Source: CAD feature listing. Evaluate the final solid. Frame: model axes, mm. Face numbers are marked on the shaded views. A direction names the side the tool comes from. Give positions to 0.01 mm unless a question says otherwise; leave off trailing zeros. Loops run counter-clockwise (first coordinate to the right, second up) from the corner with the lowest first, then second, coordinate; pieces in that order, holes last. Notation, with made-up numbers: M -25.75,-32 L 17.25,-32 A14 ccw 17.25,-5 Z; hole C -3.5,13.25 d5. An arc over 180 degrees is marked long. Answer in a Markdown table with one row per item.
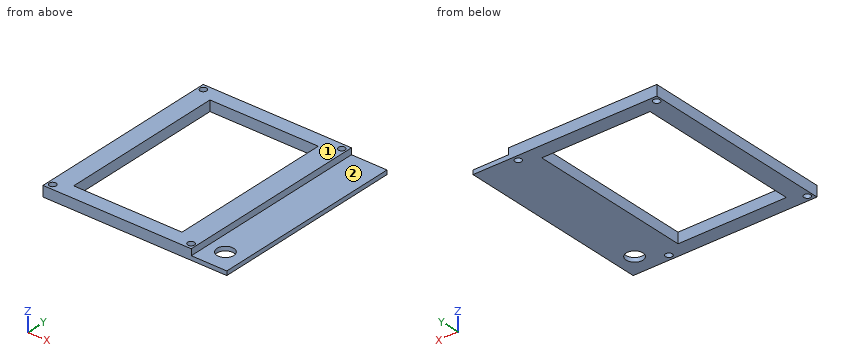
```python
from build123d import *

# Parameters (mm, degrees)
SKETCH_1_W          = 71
SKETCH_1_H          = 93
SKETCH_1_R          = 1.6
SKETCH_1_W_2        = 51
SKETCH_1_H_2        = 78.2
EXTRUDE_1_DEPTH     = 5
SKETCH_2_W          = 71
SKETCH_2_H          = 93
SKETCH_2_W_2        = 70.5
SKETCH_2_H_2        = 92.5
CUT_EXTRUDE_1_DEPTH = 6
SKETCH_3_W          = 51.5
SKETCH_3_H          = 78.7
SKETCH_3_W_2        = 51
SKETCH_3_H_2        = 78.2
CUT_EXTRUDE_2_DEPTH = 6
SKETCH_5_W          = 27
SKETCH_5_H          = 92.5
SKETCH_5_R          = 1.6
EXTRUDE_3_DEPTH     = 2
SKETCH_7_R          = 4
CUT_EXTRUDE_3_DEPTH = 6


with BuildPart() as part:
    # Эскиз1 → Бобышка-Вытянуть1 (new body)
    with BuildSketch(Plane(origin=(0, 0, 92.662297423), x_dir=(-1, 0, 0), z_dir=(0, 0, -1))):
        with Locations((-39.5, 51)):
            Rectangle(SKETCH_1_W, SKETCH_1_H)
        with Locations((-6.6, 7.5)):
            Circle(SKETCH_1_R, mode=Mode.SUBTRACT)
        with Locations((-72.4, 7.5)):
            Circle(SKETCH_1_R, mode=Mode.SUBTRACT)
        with Locations((-6.6, 94.5)):
            Circle(SKETCH_1_R, mode=Mode.SUBTRACT)
        with Locations((-72.4, 94.5)):
            Circle(SKETCH_1_R, mode=Mode.SUBTRACT)
        with Locations((-38.9, 51)):
            Rectangle(SKETCH_1_W_2, SKETCH_1_H_2, mode=Mode.SUBTRACT)
    extrude(amount=EXTRUDE_1_DEPTH)

    # Эскиз2 → Вырез-Вытянуть1 (cut, through all)
    with BuildSketch(Plane.XY.offset(92.662297423)):
        with Locations((39.5, 51)):
            Rectangle(SKETCH_2_W, SKETCH_2_H)
        with Locations((39.5, 51)):
            Rectangle(SKETCH_2_W_2, SKETCH_2_H_2, mode=Mode.SUBTRACT)
    extrude(amount=-CUT_EXTRUDE_1_DEPTH, mode=Mode.SUBTRACT)

    # Эскиз3 → Вырез-Вытянуть2 (cut, through all)
    with BuildSketch(Plane.XY.offset(92.662297423)):
        with Locations((38.9, 51)):
            Rectangle(SKETCH_3_W, SKETCH_3_H)
        with Locations((38.9, 51)):
            Rectangle(SKETCH_3_W_2, SKETCH_3_H_2, mode=Mode.SUBTRACT)
    extrude(amount=-CUT_EXTRUDE_2_DEPTH, mode=Mode.SUBTRACT)

    # Эскиз5 → Бобышка-Вытянуть3 (add)
    with BuildSketch(Plane(origin=(0, 0, 87.662297423), x_dir=(-1, 0, 0), z_dir=(0, 0, -1))):
        with Locations((-78.15, 51)):
            Rectangle(SKETCH_5_W, SKETCH_5_H)
        with Locations((-72.4, 94.5)):
            Circle(SKETCH_5_R, mode=Mode.SUBTRACT)
        with Locations((-72.4, 7.5)):
            Circle(SKETCH_5_R, mode=Mode.SUBTRACT)
    extrude(amount=-EXTRUDE_3_DEPTH)

    # Эскиз7 → Вырез-Вытянуть3 (cut, through all)
    with BuildSketch(Plane(origin=(0, 0, 87.662297423), x_dir=(-1, 0, 0), z_dir=(0, 0, -1))):
        with Locations((-82.7, 14.8)):
            Circle(SKETCH_7_R)
    extrude(amount=-CUT_EXTRUDE_3_DEPTH, mode=Mode.SUBTRACT)


solid = part.part
```
1) Set-up query: the marked faces 1 and 2. Return all of +Z, -Z, +X, -X, +Y, -Y with unobstructed straight access to the full face (end or side cutting, diameter ignored); none if empty.
Reply:
| item | result |
|---|---|
| face 1 | +Z, +X, -X, +Y, -Y |
| face 2 | +Z, +X, +Y, -Y |
2) Section D-D, the plane x = 72.4. Return loops of the section in (y, z).
Reply:
| item | result |
|---|---|
| outline | M 4.75,87.66 L 5.9,87.66 L 5.9,92.66 L 4.75,92.66 Z; M 9.1,87.66 L 92.9,87.66 L 92.9,92.66 L 9.1,92.66 Z; M 96.1,87.66 L 97.25,87.66 L 97.25,92.66 L 96.1,92.66 Z |
3) Section B-B, the plane y = 7.5. Return loops of the section in (x, z), then the cut area to 3 significant figures.
Reply:
| item | result |
|---|---|
| outline | M 4.25,87.66 L 5,87.66 L 5,92.66 L 4.25,92.66 Z; M 8.2,87.66 L 70.8,87.66 L 70.8,92.66 L 8.2,92.66 Z; M 74,87.66 L 91.65,87.66 L 91.65,89.66 L 74.75,89.66 L 74.75,92.66 L 74,92.66 Z |
| area | 354 mm² |
4) Material intervals for L1, parallel to X at y = 94.5, z = 91.2; L2, parallel to Y at x = 6.6, z = 90.15; L3, parallel to X at y = 39, z = 90.6, sorted ascending.
Reply:
| item | result |
|---|---|
| L1 | x = 4.25 to 5, 8.2 to 70.8, 74 to 74.75 |
| L2 | y = 4.75 to 5.9, 9.1 to 92.9, 96.1 to 97.25 |
| L3 | x = 4.25 to 13.15, 64.65 to 74.75 |
5) Section A-A, the plane x = 18.5. Return loops of the section in (y, z), then the cut area to 3 significant figures.
Reply:
| item | result |
|---|---|
| outline | M 4.75,87.66 L 11.65,87.66 L 11.65,92.66 L 4.75,92.66 Z; M 90.35,87.66 L 97.25,87.66 L 97.25,92.66 L 90.35,92.66 Z |
| area | 69.0 mm² |
6) Section C-C, the plane z = 88.45. Return loops of the section in (x, y).
Reply:
| item | result |
|---|---|
| outline | M 4.25,4.75 L 91.65,4.75 L 91.65,97.25 L 4.25,97.25 Z; hole C 6.6,7.5 d3.2; hole C 6.6,94.5 d3.2; hole M 13.15,11.65 L 64.65,11.65 L 64.65,90.35 L 13.15,90.35 Z; hole C 72.4,7.5 d3.2; hole C 72.4,94.5 d3.2; hole C 82.7,14.8 d8 |
7) Pin query (flat end, axial travel): pin 1 Ø4 at (x, y) = (72.4, 94.5) entering from -Z; pin 2 Ø5 at (x, y) = (83.5, 57) entering from +Z; pin 3 Ø0.9 at (y, z) = (71.5, 92) entering from +X. Return the tip coordinate at first contact, or that it passes through.
Reply:
| item | result |
|---|---|
| pin 1 | stops at z = 87.66 |
| pin 2 | stops at z = 89.66 |
| pin 3 | stops at x = 74.75 |
